Check sheet for the modelled part. Datum: model origin and axes. Units: mm. A direction names the side the tool comes from. Round coordinates to 2 decimals unless told otherwise and drop trailing zeros. Loops run counter-clockwise (first coordinate to the right, second up) from the corner with the lowest first, then second, coordinate; pieces in that order, holes last. Notation, with made-up numbers: (-25.5, 21) -> (-14.5, 21) arc R23 cw to (-14.5, 36) -> close; hole circle Ø9 at (35, 50). An arc over 180 degrees is marked (long way). Use one line per item in the form item = value. Start each with the question number.
(1) Material ranges on probe 1 along Z at (x, y) = (0, 21); probe 2 along X at (y, z) = (20.75, 0); probe 3 along Y at (x, z) = (-11, -41.5), recorded low to high. Write a range as [from, to].
(2) Sectioned sample at B-B (y = 3.5). State how many separate pieces and enclosed holes the cut face has, and give its area (3 significant figures).
(3) Draft check along Z on faces 4 (the flat face through (0, -3, -48)), 5 (the flat face through (0, -11, -47)), 6 (the flat face through (0, 14, -65)), 7 (the cylindrical face through (0.275, 13.804, 12.497)). Enter one of: released by +Z, released by -Z, zero draft, split by the parting line, or undercut.
(4) Sectioned sample at D-D (z = -1.5). Record the cut outline in (x, y), and give its area (3 significant figures).
(5) Sectioned sample at A-A (z = -54). Record the cut outline in (x, y), and give its area (3 significant figures).
(6) Set-up check for faces 1 (the flat face through (0, 31, -47)), 2 (the flat face through (0, 28, -11)), 3 (the flat face through (-12.5, 14, -10)): record each of +Z, -Z, +X, -X, +Y, -Y from which the full face is reachable in a straight line by a thin tool's end or side.
(7) Go/stop test with flat-tipped pins: pin 1 (1.5 mm diameter, centred on y = 1, z = -19, fed in from -X); pin 2 (16 mm diameter, centred on y = 9.5, z = -14.5, fed in from -X) (3 decimals); pin 3 (16 mm diameter, centred on y = 18, z = -11.5, fed in from +X); pin 4 (8 mm diameter, centred on x = 3, y = 23, fed in from +Z). Record where each tip stops, or that it passes through.
Autodesk Inventor part; units mm, degrees
ref_plane "YZ Plane" through (0, 0, 0) normal (1, 0, 0) x (0, 1, 0)
ref_plane "XZ Plane" through (0, 0, 0) normal (0, 1, 0) x (-1, 0, 0)
sketch "Sketch1" plane through (0, 0, 0) normal (0, 1, 0) x (-1, 0, 0)
  circle A0 centre (0, 0) radius 10
  circle A1 centre (0, 0) radius 12.5
  dimension "d0" = 20
  dimension "d1" = 25
extrude "Extrusion1" add sketch "Sketch1" along normal blind 28
sketch "Sketch2" plane through (0, 0, 0) normal (0, 0, 1) x (1, 0, 0)
  line L0 (12.5, 0) -> (-12.5, 0)
  line L1 (12.5, 28) -> (-12.5, 28)
  line L2 (-12.5, 0) -> (12.5, 0)
  line L3 (12.5, 0) -> (12.5, 28)
  line L4 (12.5, 28) -> (-12.5, 28)
  line L5 (-12.5, 28) -> (-12.5, 0)
  point P0 (0, 0)
extrude "Extrusion2" add sketch "Sketch2" against normal blind 20
sketch "Sketch3" plane through (0, 28, 0) normal (0, 1, 0) x (1, 0, 0)
  circle A0 centre (0, 0) radius 10
extrude "Extrusion3" cut sketch "Sketch3" against normal blind 50
ref_plane "Work Plane1" through (0, 0, -30) normal (0, 0, -1) x (-1, 0, 0)
sketch "Sketch4" plane through (0, 0, -30) normal (0, 0, -1) x (-1, 0, 0)
  line L0 (0, 0) -> (0, 28)
  line L1 (12.5, 28) -> (-12.5, 28)
  line L2 (-15, 30) -> (15, 30)
  line L3 (15, 30) -> (15, -2)
  line L4 (15, -2) -> (-15, -2)
  line L5 (-15, -2) -> (-15, 30)
  line L6 (-15, 30) -> (15, -2) construction
  line L7 (15, 30) -> (-15, -2) construction
  point P0 (0, 14)
  dimension "d9" = 30
  dimension "d10" = 32
extrude "Extrusion4" add sketch "Sketch4" along normal blind 15
sketch "Sketch5" plane through (0, 0, -45) normal (0, 0, -1) x (-1, 0, 0)
  line L0 (15, 30) -> (-15, 30)
  line L1 (0, 30) -> (0, -2)
  line L2 (-15, -2) -> (15, -2)
  line L3 (-15, 39) -> (15, 39)
  line L4 (15, 39) -> (15, -11)
  line L5 (15, -11) -> (-15, -11)
  line L6 (-15, -11) -> (-15, 39)
  line L7 (-15, 39) -> (15, -11) construction
  line L8 (15, 39) -> (-15, -11) construction
  point P0 (0, 0)
  point P1 (0, 14)
  dimension "d17" = 30
  dimension "d18" = 50
extrude "Extrusion5" add sketch "Sketch5" along normal blind 20 and the other way blind 15
sketch "Sketch7" plane through (15, -11, -30) normal (1, 0, 0) x (0, 0, -1)
  line L0 (0, 0) -> (35, 0)
  line L1 (17.5, 0) -> (17.5, 50)
  line L2 (35, 50) -> (0, 50)
  line L3 (35, 0) -> (35, 50)
  line L4 (35, 25) -> (0, 25)
  line L5 (0, 0) -> (0, 50)
  line L6 (7.5, 42) -> (27.5, 42)
  line L7 (27.5, 42) -> (27.5, 8)
  line L8 (27.5, 8) -> (7.5, 8)
  line L9 (7.5, 8) -> (7.5, 42)
  line L10 (7.5, 42) -> (27.5, 8) construction
  line L11 (27.5, 42) -> (7.5, 8) construction
  line L12 (27.5, 42) -> (7.5, 42)
  line L13 (7.5, 42) -> (7.5, 8)
  line L14 (7.5, 8) -> (27.5, 8)
  line L15 (27.5, 8) -> (27.5, 42)
  point P0 (-30, 11)
  point P1 (17.5, 25)
  dimension "d23" = 20
  dimension "d24" = 34
extrude "Extrusion6" cut sketch "Sketch7" against normal blind 30 contours L8 L9 L4 L1 | L1 L4 L7 L8 | L9 L6 L1 L4 | L1 L6 L7 L4
loft "Loft2" add section 1 edges at (0, 28, -20) (12.5, 14, -20) (0, 0, -20) (-12.5, 14, -20) section 2 edges at (15, 14, -30) (0, 39, -30) (-15, 14, -30) (0, -11, -30)
equation "\"BendRadius\" = Thickness"
equation "\"BendReliefWidth\" = Thickness"
equation "\"BendReliefDepth\" = 0.5 * Thickness"
equation "\"CornerReliefSize\" = 4 * Thickness"
equation "\"MinimumRemnant\" = 2 * Thickness"
equation "\"TransitionRadius\" = BendRadius"
equation "\"JacobiRadiusSize\" = BendRadius"
equation "\"GapSize\" = Thickness"
Checks:
q1.probe_1 = [-65, -57.5], [-37.5, -10], [10, 12.5]
q1.probe_2 = [-12.5, -10], [10, 12.5]
q1.probe_3 = [-11, -3], [31, 39]
q2.separate_pieces = 2
q2.enclosed_holes = 1
q2.area = 1,160 mm2
q3.face_4 = undercut
q3.face_5 = zero draft
q3.face_6 = released by -Z
q3.face_7 = released by +Z
q4.outline = (-12.5, 0) -> (-9.89, 0) -> (-9.89, 28) -> (-12.5, 28) -> close; (9.89, 0) -> (12.5, 0) -> (12.5, 28) -> (9.89, 28) -> close
q4.area = 146 mm2
q5.outline = (-15, -11) -> (15, -11) -> (15, -3) -> (-15, -3) -> close; (-15, 31) -> (15, 31) -> (15, 39) -> (-15, 39) -> close
q5.area = 480 mm2
q6.face_1 = +X, -X
q6.face_2 = +Z, +X, -X, +Y
q6.face_3 = +Z, -X, +Y, -Y
q7.pin_1 = -12.5
q7.pin_2 = -13.125
q7.pin_3 = 12.5
q7.pin_4 = 12.5
